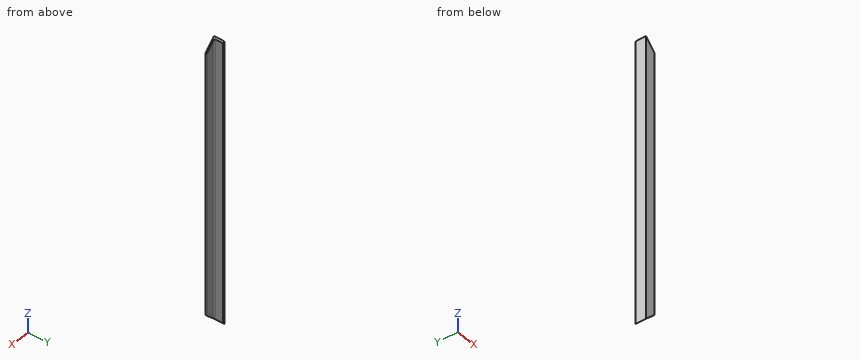
Autodesk Inventor part; units mm, degrees
ref_plane "Start Plane" through (0, 0, 0) normal (0, 0, 1) x (1, 0, 0)
ref_plane "End Plane" through (0, 0, 690) normal (0, 0, 1) x (1, 0, 0)
ref_plane "Work Plane4" through (0, 12.7, 0) normal (0.7071, 0, -0.7071) x (-0.7071, 0, -0.7071)
ref_plane "Start Plane" through (0, 0, 0) normal (0, 0, 1) x (1, 0, 0)
ref_plane "End Plane" through (0, 0, 690) normal (0, 0, 1) x (1, 0, 0)
sketch "Sketch" plane through (0, 0, 0) normal (0, 0, 1) x (1, 0, 0)
  line L0 (25.4, 0) -> (0, 0)
  line L1 (0, 0) -> (0, 25.4)
  line L2 (0, 25.4) -> (1.651, 25.4)
  line L3 (3.175, 23.876) -> (3.175, 6.477)
  line L4 (6.477, 3.175) -> (23.876, 3.175)
  line L5 (25.4, 1.651) -> (25.4, 0)
  line L6 (0, -11.0414) -> (0, 31.5385) construction
  line L7 (-11.0414, 0) -> (31.5385, 0) construction
  arc A0 (3.175, 6.477) -> (6.477, 3.175) centre (6.477, 6.477) ccw
  arc A1 (3.175, 23.876) -> (1.651, 25.4) centre (1.651, 23.876) ccw
  arc A2 (25.4, 1.651) -> (23.876, 3.175) centre (23.876, 1.651) ccw
  line L8 (0, 40.0545) -> (0, -19.5574) construction
  line L9 (-19.5574, 0) -> (40.0545, 0) construction
  point P0 (3.175, 25.4)
  point P1 (3.175, 3.175)
  point P2 (25.4, 3.175)
  dimension "d0" = 25.4
  dimension "d1" = 25.4
  dimension "d2" = 3.175
  dimension "d3" = 3.175
  dimension "d10" = 0
  dimension "d11" = 0
  dimension "d14" = 3.302
  dimension "d15" = 1.524
extrude "Body" add sketch "Sketch" along normal up to surface (690 mm away) from surface at 0
sketch "Sketch3" plane through (0, 0, 0) normal (0, 0, 1) x (1, 0, 0)
  line L0 (0, 0) -> (10, 0)
ref_plane "Work Plane3" through (0, 0, 0) normal (0, -1, 0) x (1, 0, 0)
ref_plane "Work Plane4" through (0, 12.7, 0) normal (0.7071, 0, -0.7071) x (-0.7071, 0, -0.7071)
split "Split1" plane through (0, 12.7, 0) removes the side toward (0.7071, 0, -0.7071)
ref_plane "Work Plane5" through (0, 12.7, 690) normal (0.7071, 0, 0.7071) x (0.7071, 0, -0.7071)
split "Split2" plane through (0, 12.7, 690) removes the side toward (0.7071, 0, 0.7071)
sketch "Sketch4" plane through (0, 0, 0) normal (0, -1, 0) x (1, 0, 0)
  line L0 (-2, 0) -> (12, 0)
  line L1 (-2, 690) -> (12, 690)
  dimension "d17" = 690
equation "\"d0\" = G_H"
equation "\"d1\" = G_H"
equation "\"d2\" = G_T"
equation "\"d3\" = G_T"
equation "\"d14\" = G_IR"
equation "\"d15\" = G_ER"
equation "\"d4\" = G_L"
equation "\"G_H\" = 25.4"
equation "\"G_T\" = 3.175"
equation "\"G_ER\" = 1.524"
equation "\"G_IR\" = 3.302"
equation "\"G_L\" = d17"
equation "\"ex\" = 0"
equation "\"G_OFFSET_START\" = 0"
equation "\"G_OFFSET_END\" = 0"
equation "\"d13\" = G_OFFSET_END + B_L"
equation "\"B_L\" = 690"
properties part number "AISC - L 1 x 1 x 1/8 - 27.165" material "Steel, Mild"
Part model, mm, in its own coordinate system. Coordinates: 2 decimals unless noted, no trailing zeros. Order: outer loops, then holes, each group sorted by start corner. A loop starts at its lowest first (then second) coordinate and runs counter-clockwise, first axis right, second up. Notation, with made-up numbers: M 6.25,6 L 32.25,6 A6 ccw 32.25,16 Z; hole C 68.5,-16 d4. An arc over 180 degrees is marked long. Use a Markdown table: item, result.
(1) Probe L1, parallel to Y at x = 22.5, z = 622 (3 decimals); L2, parallel to Y at x = 2, z = 385. List the from-to ranges inside material, lowest first.
A:
| item | result |
|---|---|
| L1 | y = 0 to 3.175 |
| L2 | y = 0 to 25.36 |
(2) Cut at B-B on x = 17.25. Write the cut outline in (y, z) (3 decimals).
A:
| item | result |
|---|---|
| outline | M 0,17.25 L 3.175,17.25 L 3.175,672.75 L 0,672.75 Z |
(3) Flat gauge pins, fed straight in: pin 1 (5 mm diameter, centred on x = 4, y = 10.5, fed in from -Z); pin 2 (4 mm diameter, centred on x = 4.5, y = 16.5, fed in from +Z); pin 3 (10 mm diameter, centred on x = 7, y = 12.5, fed in from -Z). Where does each tip first touch, or does it go through?
A:
| item | result |
|---|---|
| pin 1 | stops at z = 1.5 |
| pin 2 | stops at z = 687.5 |
| pin 3 | stops at z = 2 |
(4) Cut at C-C on y = 17. Write the cut outline in (x, z) (3 decimals).
A:
| item | result |
|---|---|
| outline | M 0,0 L 3.175,3.175 L 3.175,686.825 L 0,690 Z |
(5) Cut at A-A on z = 77. Write the cut outline in (x, y) (3 decimals).
A:
| item | result |
|---|---|
| outline | M 0,0 L 25.4,0 L 25.4,1.651 A1.524 ccw 23.876,3.175 L 6.477,3.175 A3.302 cw 3.175,6.477 L 3.175,23.876 A1.524 ccw 1.651,25.4 L 0,25.4 Z |
